Source: CAD feature listing. Evaluate the final solid. Frame: model axes, mm. Face numbers are marked on the shaded views. A direction names the side the tool comes from. Give positions to 0.01 mm unless a question says otherwise; leave off trailing zeros. Order: outer loops, then holes, each group sorted by start corner. A loop starts at its lowest first (then second) coordinate and runs counter-clockwise, first axis right, second up.
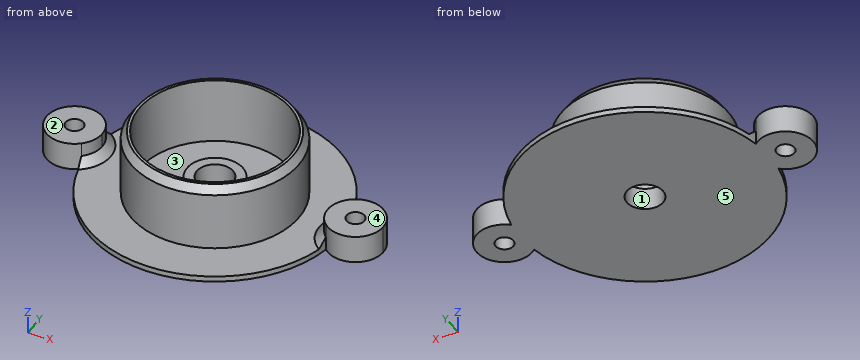
from build123d import *

# Parameters (mm, degrees)
F0_R         = 1.6
F1_DEPTH     = 5
F2_DEPTH     = 1
F3_R         = 15
F3_R_2       = 13.5
F4_DEPTH     = 12
F5_SIZE2     = 1.5
F5_SIZE      = 1
F8_T4_ANGLE  = 185.4300536725
F8_S5_R      = 22.5
F8_T6_DEPTH  = 9
F8_T10_ANGLE = 185.4300536725
F8_S11_R     = 22.5
F8_T12_DEPTH = 9
F9_R         = 5
F10_DEPTH    = 3
F11_R        = 3.25
F12_DEPTH    = 5


# Not quite as in the source:
# - a fillet or chamfer that OpenCascade refuses, or shapes differently, is made with other operations: its cross-section is extruded or revolved along the edge and cut away or added
# - a feature of the source that left no trace in its solid (it failed there, or was rolled back) is left out


with BuildPart() as f1:
    # F0 (on Top) → F1 (new body)
    with BuildSketch(Plane.XY):
        with BuildLine():
            ThreePointArc((-22.1862745098, -3.7442253372), (-22.5, 0), (-22.1862745098, 3.7442253372))
            ThreePointArc((-22.1862745098, 3.7442253372), (-30.5, 0), (-22.1862745098, -3.7442253372))
        make_face()
        with Locations((-25.5, 0)):
            Circle(F0_R, mode=Mode.SUBTRACT)
        with BuildLine():
            ThreePointArc((-20.5, 0), (-20.9410183456, 2.0532136456), (-22.1862745098, 3.7442253372))
            ThreePointArc((-22.1862745098, 3.7442253372), (-22.5, 0), (-22.1862745098, -3.7442253372))
            ThreePointArc((-22.1862745098, -3.7442253372), (-20.9410183456, -2.0532136456), (-20.5, 0))
        make_face()
    extrude(amount=F1_DEPTH)



with BuildPart() as f1b:
    # F0 (on Top) → F1, piece 2 (new body)
    with BuildSketch(Plane.XY):
        with BuildLine():
            ThreePointArc((22.1862745098, 3.7442253372), (22.4214314493, 1.8786728733), (22.5, 0))
            ThreePointArc((22.5, 0), (22.4214314493, -1.8786728733), (22.1862745098, -3.7442253372))
            ThreePointArc((22.1862745098, -3.7442253372), (27.5532136456, -4.5589816544), (30.5, 0))
            ThreePointArc((30.5, 0), (27.5532136456, 4.5589816544), (22.1862745098, 3.7442253372))
        make_face()
        with Locations((25.5, 0)):
            Circle(F0_R, mode=Mode.SUBTRACT)
        with BuildLine():
            ThreePointArc((22.1862745098, -3.7442253372), (22.4214314493, -1.8786728733), (22.5, 0))
            ThreePointArc((22.5, 0), (22.4214314493, 1.8786728733), (22.1862745098, 3.7442253372))
            ThreePointArc((22.1862745098, 3.7442253372), (20.5, 0), (22.1862745098, -3.7442253372))
        make_face()
    extrude(amount=F1_DEPTH)


with BuildPart() as f1_1:
    add(f1.part)

    add(f1b.part)  # F2 merges F1b
    # F0 (on Top) → F2 (join)
    with BuildSketch(Plane.XY):
        with BuildLine():
            ThreePointArc((22.1862745098, -3.7442253372), (20.5, 0), (22.1862745098, 3.7442253372))
            ThreePointArc((22.1862745098, 3.7442253372), (0, 22.5), (-22.1862745098, 3.7442253372))
            ThreePointArc((-22.1862745098, 3.7442253372), (-20.9410183456, 2.0532136456), (-20.5, 0))
            ThreePointArc((-20.5, 0), (-20.9410183456, -2.0532136456), (-22.1862745098, -3.7442253372))
            ThreePointArc((-22.1862745098, -3.7442253372), (0, -22.5), (22.1862745098, -3.7442253372))
        make_face()
    extrude(amount=F2_DEPTH)

    # F3 (on face) → F4 (join)
    with BuildSketch(Plane.XY.offset(1)):
        Circle(F3_R)
        Circle(F3_R_2, mode=Mode.SUBTRACT)
    extrude(amount=F4_DEPTH)

    # F5
    f5_edges = [f1_1.edges().sort_by_distance(p)[0] for p in [
        (-15, 0, 13),
    ]]
    f5_side = f1_1.faces().sort_by_distance((-14.575736, 0, 13))[0]
    chamfer(f5_edges, length=F5_SIZE, length2=F5_SIZE2, reference=f5_side)

    # F8: chamfer of 1.5 on 2 edges, made by hand


with BuildPart() as f8_tool2:
    # F8_s3 → F8_t4 (revolve)
    with BuildSketch(Plane(origin=(25.4427839223, 1.2065389767, 0), x_dir=(0, 0, 1), z_dir=(0.9988774861, 0.0473684257, 0))):
        Polygon((1, 7.7078948555), (2.5, 6.2078948555), (1, 6.2078948555), align=None)
    revolve(axis=Axis((25.5, 0, 1), (0, 0, -1)), revolution_arc=F8_T4_ANGLE)

    # F8_s5 → F8_t6 (intersect, symmetric)
    with BuildSketch(Plane.XY.offset(1.8)):
        Circle(F8_S5_R)
    extrude(amount=F8_T6_DEPTH, both=True, mode=Mode.INTERSECT)


with BuildPart() as f1_2:
    add(f1_1.part)

    # F8_t1: union F8_tool2
    add(f8_tool2.part)


with BuildPart() as f8_tool8:
    # F8_s9 → F8_t10 (revolve)
    with BuildSketch(Plane(origin=(-25.4427839223, 1.2065389767, 0), x_dir=(0, 0, 1), z_dir=(-0.9988774861, 0.0473684257, 0))):
        Polygon((1, -7.7078948555), (2.5, -6.2078948555), (1, -6.2078948555), align=None)
    revolve(axis=Axis((-25.5, 0, 1), (0, 0, 1)), revolution_arc=F8_T10_ANGLE)

    # F8_s11 → F8_t12 (intersect, symmetric)
    with BuildSketch(Plane.XY.offset(1.7)):
        Circle(F8_S11_R)
    extrude(amount=F8_T12_DEPTH, both=True, mode=Mode.INTERSECT)


with BuildPart() as f1_3:
    add(f1_2.part)

    # F8_t7: union F8_tool8
    add(f8_tool8.part)

    # F9 (on face) → F10 (join)
    with BuildSketch(Plane.XY.offset(1)):
        Circle(F9_R)
    extrude(amount=F10_DEPTH)

    # F11 (on face) → F12 (cut)
    with BuildSketch(Plane.XY.offset(4)):
        Circle(F11_R)
    extrude(amount=-F12_DEPTH, mode=Mode.SUBTRACT)


solid = f1_3.part
(1) Line query: line 1 along Y through (x, z) = (0, 2.45); line 2 along Y through (x, z) = (25.5, 2.3); line 3 along X through (y, z) = (2.5, 3.75). Output: solid intervals per line, ascending.
(2) Section B-B, the plane z = 6.75. Return loops of the section in (x, y), plus the area to 3 significant figures.
(3) Section D-D, the plane y = -19. Return loops of the section in (x, z).
(4) Draft query along X for the marked faces 1 and 2. Return one class per face: +X half, -X half, draft (parallel to the pull), parting line (faces both ways), or undercut.
(5) Section C-C, the plane x = -25.5. Return loops of the section in (y, z), plus the area to 3 significant figures.
(6) Access query for the marked faces 3, 4 and 5. Directions: +Z, -Z, +X, -X, +Y, -Y. A direction counts if a zero-diameter tool reaches every point of the face in a straight line with its end or side. Return the directions, or none.
(7) Pin query (flat end, axial travel): pin 1 Ø8 at (x, y) = (-23, 0) entering from +Z; pin 2 Ø5 at (x, y) = (0.5, 1) entering from +Z; pin 3 Ø5 at (y, z) = (-3, 8.5) entering from -X. Return the tip coordinate at first contact, or that it passes through.
(8) Section A-A, the plane x = 0. Return loops of the section in (y, z).
Checks:
1. line 1: y = -15 to -13.5, -5 to -3.25, 3.25 to 5, 13.5 to 15
1. line 2: y = -5 to -1.6, 1.6 to 5
1. line 3: x = -29.83 to -21.17, -14.79 to -13.27, -4.33 to -2.08, 2.08 to 4.33, 13.27 to 14.79, 21.17 to 29.83
2. outline: circle Ø30 at (0, 0); hole circle Ø27 at (0, 0)
2. area: 134 mm2
3. outline: (-12.05, 0) - (12.05, 0) - (12.05, 1) - (-12.05, 1) - close
4. face 1: undercut
4. face 2: draft
5. outline: (-5, 0) - (-1.6, 0) - (-1.6, 5) - (-5, 5) - close; (1.6, 0) - (5, 0) - (5, 5) - (1.6, 5) - close
5. area: 34.0 mm2
6. face 3: +Z
6. face 4: +Z, +X, +Y, -Y
6. face 5: -Z, +X, -X, +Y, -Y
7. pin 1: stops at z = 5
7. pin 2: stops at z = 4
7. pin 3: stops at x = -14.99
8. outline: (-22.5, 0) - (-3.25, 0) - (-3.25, 4) - (-5, 4) - (-5, 1) - (-13.5, 1) - (-13.5, 13) - (-14, 13) - (-15, 11.5) - (-15, 1) - (-22.5, 1) - close; (3.25, 0) - (22.5, 0) - (22.5, 1) - (15, 1) - (15, 11.5) - (14, 13) - (13.5, 13) - (13.5, 1) - (5, 1) - (5, 4) - (3.25, 4) - close
